Check sheet for the modelled part. Datum: model origin and axes. Units: mm. A direction names the side the tool comes from. Coordinates: 2 decimals unless noted, no trailing zeros. Order: outer loops, then holes, each group sorted by start corner. A loop starts at its lowest first (then second) coordinate and runs counter-clockwise, first axis right, second up.
1. Cross-section at C-C (z = 8). Enter the section's corners in (x, y), then the cut area to 3 significant figures.
2. Set-up check for faces 1 (the cylindrical face through (0.15, 37.5, 4.93)), 2 (the flat face through (19, -15, 6)), 3 (the flat face through (7, -52, 5)): record each of +Z, -Z, +X, -X, +Y, -Y from which the full face is reachable in a straight line by a thin tool's end or side.
3. Draft check along Y on faces 4 (the flat face through (-13, 60, 5)), 5 (the flat face through (55, -37.5, 5)), 6 (the cylindrical face through (-32.4, 15.8, 3)), 7 (the flat face through (-27, -1, 10)). Enter one of: released by +Y, released by -Y, zero draft, split by the parting line, or undercut.
4. Cross-section at D-D (y = 12.5). Enter the section's corners in (x, z), then the cut area to 3 significant figures.
5. Cross-section at A-A (y = 48). Enter the section's corners in (x, z), then the cut area to 3 significant figures.
6. Cross-section at B-B (x = 17). Enter the section's corners in (y, z), then the cut area to 3 significant figures.
7. Gauge pin test, flat ends, axial feed: pin 1 Ø9.5 at (x, y) = (17, -12.5) entering from -Z; pin 2 Ø5 at (x, z) = (56.5, 3.5) entering from -Y; pin 3 Ø5.5 at (x, y) = (17, 12.5) entering from +Z; pin 4 Ø3 at (x, z) = (-66, 1.5) entering from +Y. Record the tip position at first contact, or that the pin passes through.
8. Thickness scan on line 1 (Y direction, x = 17, z = 7.9); line 2 (Y direction, x = -73, z = 6.8); line 3 (Y direction, x = 43.5, z = 6.25). Record the ranges inside material, lowest first.
```python
from build123d import *

# Parameters (mm, degrees)
F1_DEPTH       = 10
F2_D           = 6
F2_CBORE_D     = 11
F2_CBORE_DEPTH = 6


with BuildPart() as f1:
    # F0 (on Top) → F1 (new body)
    with BuildSketch(Plane.XY):
        with BuildLine():
            Line((-118, 17.5), (-118, 0))
            Line((-118, 0), (67, 0))
            Line((67, 0), (67, 37.5))
            Line((67, 37.5), (42, 37.5))
            Line((42, 37.5), (19.5, 60))
            Line((19.5, 60), (7, 60))
            Line((7, 60), (7, 44.5))
            ThreePointArc((7, 44.5), (0, 37.5), (-7, 44.5))
            Line((-7, 44.5), (-7, 60))
            Line((-7, 60), (-19.5, 60))
            Line((-19.5, 60), (-42, 37.5))
            Line((-42, 37.5), (-98, 37.5))
            Line((-98, 37.5), (-118, 17.5))
        make_face()
    extrude(amount=F1_DEPTH)

    # F2 (through all)
    with Locations(Plane(origin=(0, 0, 0), x_dir=(1, 0, 0), z_dir=(0, 0, -1))):
        with Locations((-73, -12.5), (-28, -12.5), (17, -12.5)):
            CounterBoreHole(F2_D / 2, F2_CBORE_D / 2, F2_CBORE_DEPTH)

    # F3: F1 across plane


with BuildPart() as f1_1:
    add(f1.part)
    add(f1.part.mirror(Plane.XZ))


solid = f1_1.part
```
Data:
1. outline: (-118, -17.5) - (-98, -37.5) - (-42, -37.5) - (-19.5, -60) - (-7, -60) - (-7, -44.5) arc R7 cw to (7, -44.5) - (7, -60) - (19.5, -60) - (42, -37.5) - (67, -37.5) - (67, 37.5) - (42, 37.5) - (19.5, 60) - (7, 60) - (7, 44.5) arc R7 cw to (-7, 44.5) - (-7, 60) - (-19.5, 60) - (-42, 37.5) - (-98, 37.5) - (-118, 17.5) - close; hole circle Ø6 at (-73, -12.5); hole circle Ø6 at (-73, 12.5); hole circle Ø6 at (-28, -12.5); hole circle Ø6 at (-28, 12.5); hole circle Ø6 at (17, -12.5); hole circle Ø6 at (17, 12.5)
1. area: 15,500 mm2
2. face 1: +Z, -Z, +Y
2. face 2: -Z
2. face 3: +Z, -Z, -Y
3. face 4: released by +Y
3. face 5: released by -Y
3. face 6: undercut
3. face 7: zero draft
4. outline: (-118, 0) - (-78.5, 0) - (-78.5, 6) - (-76, 6) - (-76, 10) - (-118, 10) - close; (-70, 6) - (-67.5, 6) - (-67.5, 0) - (-33.5, 0) - (-33.5, 6) - (-31, 6) - (-31, 10) - (-70, 10) - close; (-25, 6) - (-22.5, 6) - (-22.5, 0) - (11.5, 0) - (11.5, 6) - (14, 6) - (14, 10) - (-25, 10) - close; (20, 6) - (22.5, 6) - (22.5, 0) - (67, 0) - (67, 10) - (20, 10) - close
4. area: 1,580 mm2
5. outline: (-31.5, 0) - (-7, 0) - (-7, 10) - (-31.5, 10) - close; (7, 0) - (31.5, 0) - (31.5, 10) - (7, 10) - close
5. area: 490 mm2
6. outline: (-60, 0) - (-18, 0) - (-18, 6) - (-15.5, 6) - (-15.5, 10) - (-60, 10) - close; (-9.5, 6) - (-7, 6) - (-7, 0) - (7, 0) - (7, 6) - (9.5, 6) - (9.5, 10) - (-9.5, 10) - close; (15.5, 6) - (18, 6) - (18, 0) - (60, 0) - (60, 10) - (15.5, 10) - close
6. area: 1,020 mm2
7. pin 1: stops at z = 6
7. pin 2: stops at y = -37.5
7. pin 3: passes through
7. pin 4: stops at y = 37.5
8. line 1: y = -60 to -15.5, -9.5 to 9.5, 15.5 to 60
8. line 2: y = -37.5 to -15.5, -9.5 to 9.5, 15.5 to 37.5
8. line 3: y = -37.5 to 37.5
